Could you check a few things on this model? Use its own coordinates, in mm. A direction names the side the tool comes from. Give positions to 0.01 mm unless a question says otherwise; leave off trailing zeros. Loops run counter-clockwise (first coordinate to the right, second up) from the corner with the lowest first, then second, coordinate; pieces in that order, holes last. Notation, with made-up numbers: (80.5, 33.25) -> (119.5, 33.25) arc R22 cw to (119.5, 69.25) -> close; hole circle Ø6 at (67.25, 79.5). An arc over 180 degrees is marked (long way). Put each result on its own line as item: value.
```python
from build123d import *

# Parameters (mm, degrees)
SKETCH_2_W          = 10
SKETCH_2_H          = 10
SKETCH_2_W_2        = 8
SKETCH_2_H_2        = 8
EXTRUDE_1_DEPTH     = 165
SKETCH_3_R          = 1.75
SKETCH_3_R_2        = 1.5
CUT_EXTRUDE_1_DEPTH = 11


with BuildPart() as part:
    # 草图2 → 拉伸-薄壁1 (new body)
    with BuildSketch(Plane(origin=(0, 0, 0), x_dir=(0, 0, -1), z_dir=(1, 0, 0))):
        Rectangle(SKETCH_2_W, SKETCH_2_H)
        Rectangle(SKETCH_2_W_2, SKETCH_2_H_2, mode=Mode.SUBTRACT)
    extrude(amount=-EXTRUDE_1_DEPTH)

    # 草图3 → 切除-拉伸1 (cut, through all)
    with BuildSketch(Plane.XY.offset(5)):
        with Locations((-6.2, 0)):
            Circle(SKETCH_3_R)
        with Locations((-158.8, 0)):
            Circle(SKETCH_3_R)
        with Locations((-32.5, 0)):
            Circle(SKETCH_3_R_2)
        with Locations((-132.5, 0)):
            Circle(SKETCH_3_R_2)
        with Locations((-66.3, 0)):
            Circle(SKETCH_3_R)
        with Locations((-98.7, 0)):
            Circle(SKETCH_3_R)
    extrude(amount=-CUT_EXTRUDE_1_DEPTH, mode=Mode.SUBTRACT)


solid = part.part
```
1. I need wall thicknesses on line 1 (Z direction, x = -109.5, y = -1); line 2 (Y direction, x = -158.8, z = 4.7). Which ranges of each line are inside material? Lowest first, please.
Recorded:
line 1: z = -5 to -4, 4 to 5
line 2: y = -5 to -1.75, 1.75 to 5
2. Thinking about a two-plate mould opening in X: for faces 1 (the face through (0, 0.1, 4.5)), 2 (the face through (-97.031, 0.526, -4.493)), 3 (the face through (-81, 0, -4)), which applies, pulls with the +X half, pulls with the -X half, needs draft (parallel to the pull), parting line crosses it, or undercut?
Recorded:
face 1: pulls with the +X half
face 2: undercut
face 3: needs draft
3. If we section it at A-A (x = -98.7): List the corners of the cut face in (y, z) for me.
Recorded:
outline: (-5, -5) -> (-1.75, -5) -> (-1.75, -4) -> (-4, -4) -> (-4, 4) -> (-1.75, 4) -> (-1.75, 5) -> (-5, 5) -> close; (1.75, -5) -> (5, -5) -> (5, 5) -> (1.75, 5) -> (1.75, 4) -> (4, 4) -> (4, -4) -> (1.75, -4) -> close
4. For faces 4 (the face through (-33.7, -0.9, 4.5)), 5 (the face through (-81, 4, 0)), which set-ups out of +Z, -Z, +X, -X, +Y, -Y let a thin tool reach every point of the face, with its end or its side?
Recorded:
face 4: +Z, -Z
face 5: +X, -X
5. If we section it at C-C (x = -132.5): List the corners of the cut face in (y, z) for me.
Recorded:
outline: (-5, -5) -> (-1.5, -5) -> (-1.5, -4) -> (-4, -4) -> (-4, 4) -> (-1.5, 4) -> (-1.5, 5) -> (-5, 5) -> close; (1.5, -5) -> (5, -5) -> (5, 5) -> (1.5, 5) -> (1.5, 4) -> (4, 4) -> (4, -4) -> (1.5, -4) -> close
6. If we section it at B-B (z = 1.75): List the corners of the cut face in (x, y) for me.
Recorded:
outline: (-165, -5) -> (0, -5) -> (0, -4) -> (-165, -4) -> close; (-165, 4) -> (0, 4) -> (0, 5) -> (-165, 5) -> close
